```python
from build123d import *

# Parameters (mm, degrees)
BOSS_EXTRUDE1_DEPTH = 3


with BuildPart() as part:
    # Sketch1 → Boss-Extrude1 (new body)
    with BuildSketch(Plane.XY):
        Polygon((70.190369541, 52.74356103), (70.190369541, 55.74356103), (50.190369541, 55.74356103), (50.190369541, 52.74356103), (30.190369541, 52.74356103), (30.190369541, 55.74356103), (10.190369541, 55.74356103), (10.190369541, 52.74356103), (-9.809630459, 52.74356103), (-9.809630459, 55.74356103), (-29.809630459, 55.74356103), (-29.809630459, 52.74356103), (-49.809630459, 52.74356103), (-49.809630459, 55.74356103), (-69.809630459, 55.74356103), (-69.809630459, 52.74356103), (-89.809630459, 52.74356103), (-92.809630459, 52.74356103), (-92.809630459, 32.74356103), (-89.809630459, 32.74356103), (-89.809630459, 12.74356103), (-92.809630459, 12.74356103), (-92.809630459, -7.25643897), (-89.809630459, -7.25643897), (-89.809630459, -27.25643897), (-92.809630459, -27.25643897), (-92.809630459, -47.25643897), (-89.809630459, -47.25643897), (-89.809630459, -50.25643897), (-69.809630459, -50.25643897), (-69.809630459, -47.25643897), (-49.809630459, -47.25643897), (-49.809630459, -50.25643897), (-29.809630459, -50.25643897), (-29.809630459, -47.25643897), (-9.809630459, -47.25643897), (-9.809630459, -50.25643897), (10.190369541, -50.25643897), (10.190369541, -47.25643897), (30.190369541, -47.25643897), (30.190369541, -50.25643897), (50.190369541, -50.25643897), (50.190369541, -47.25643897), (70.190369541, -47.25643897), (70.190369541, -50.25643897), (90.190369541, -50.25643897), (90.190369541, -47.25643897), (110.190369541, -47.25643897), (113.190369541, -47.25643897), (113.190369541, -27.25643897), (110.190369541, -27.25643897), (110.190369541, -7.25643897), (113.190369541, -7.25643897), (113.190369541, 12.74356103), (110.190369541, 12.74356103), (110.190369541, 32.74356103), (113.190369541, 32.74356103), (113.190369541, 52.74356103), (110.190369541, 52.74356103), (110.190369541, 55.74356103), (90.190369541, 55.74356103), (90.190369541, 52.74356103), align=None)
    extrude(amount=BOSS_EXTRUDE1_DEPTH)


solid = part.part
```
Work out the finished part from the listing and answer in its coordinate system (mm). Give positions to 0.01 mm unless a question says otherwise; leave off trailing zeros. Loops run counter-clockwise (first coordinate to the right, second up) from the corner with the lowest first, then second, coordinate; pieces in that order, holes last. Notation, with made-up numbers: (82, 81.5) - (117, 81.5) arc R30 cw to (117, 105.5) - close; hole circle Ø5 at (-30, 63.5). An arc over 180 degrees is marked (long way). One line per question, with ' | ' between items.
(1) The part is cut by section A-A (x = 96). Write down the section's boundary in (y, z), then the cut area to 3 significant figures.
Recorded:
outline: (-47.26, 0) - (55.74, 0) - (55.74, 3) - (-47.26, 3) - close | area: 309 mm²
(2) Straight lines are drawn through the part: probe 1 along Y at (x, z) = (-14, 0.9); probe 2 along Y at (x, z) = (33, 1.6); probe 3 along X at (y, z) = (32.5, 0.3). For each, find the intervals that lie inside material, in ascending order.
Recorded:
probe 1: y = -47.26 to 55.74 | probe 2: y = -50.26 to 52.74 | probe 3: x = -89.81 to 110.19
(3) Each of these flat-tipped pins is pushed along its axis until it touches: pin 1 Ø0.9 at (y, z) = (-15.5, 1) entering from +X; pin 2 Ø1.5 at (y, z) = (-49.5, 1) entering from +X; pin 3 Ø0.9 at (x, z) = (77, 1.5) entering from +Y. Where does it stop, or does it pass through?
Recorded:
pin 1: stops at x = 110.19 | pin 2: stops at x = 90.19 | pin 3: stops at y = 52.74
